Geometry: final body of the model. Coordinates: model frame, mm. Face numbers are marked on the shaded views. Round coordinates to 2 decimals unless told otherwise and drop trailing zeros. Write each loop counter-clockwise with the first axis right and the second up, starting at its lowest first coordinate (ties: lowest second). Pieces come first, ordered by that corner, then holes. Notation, with made-up numbers: (79, 2) - (97, 2) arc R28 ccw to (97, 33) - close; hole circle Ø9 at (23, -2). An arc over 180 degrees is marked (long way). Write each question's results on one line, items separated by ' | '.
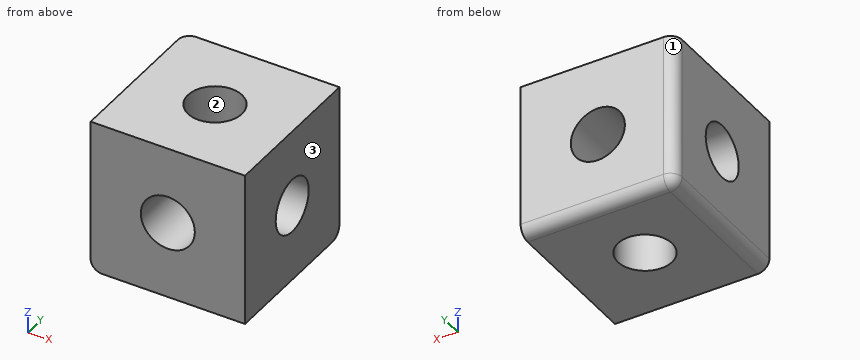
Autodesk Inventor part; units mm, degrees
ref_plane "YZ Plane" through (0, 0, 0) normal (1, 0, 0) x (0, 1, 0)
ref_plane "XZ Plane" through (0, 0, 0) normal (0, 1, 0) x (-1, 0, 0)
ref_plane "XY Plane" through (0, 0, 0) normal (0, 0, 1) x (1, 0, 0)
sketch "Sketch1" plane through (0, 0, 0) normal (0, 0, 1) x (1, 0, 0)
  line L0 (0, 0) -> (20, 0)
  line L1 (20, 0) -> (20, 20)
  line L2 (20, 20) -> (0, 20)
  line L3 (0, 20) -> (0, 0)
  circle A0 centre (10, 10) radius 3.5
  dimension "d0" = 20
  dimension "d1" = 20
  dimension "d2" = 7
extrude "Extrusion1" add sketch "Sketch1" along normal blind 20
sketch "Sketch2" plane through (20, 0, 0) normal (1, 0, 0) x (0, 0, -1)
  circle A0 centre (-10, 10) radius 3.5
  dimension "d5" = 7
extrude "Extrusion2" cut sketch "Sketch2" against normal blind 20
sketch "Sketch3" plane through (0, 0, 0) normal (0, -1, 0) x (1, 0, 0)
  circle A0 centre (10, 10) radius 3.5
  dimension "d8" = 7
extrude "Extrusion3" cut sketch "Sketch3" against normal blind 20
fillet "Fillet1" radius 1.5 3 edges at (0, 10, 0) (0, 20, 10) (10, 20, 0)
properties part number "Corner Profile"
Q1. Section query C-C, the plane y = 3.5. Return loops of the section in (x, z).
Answer block:
outline: (0, 1.5) arc R1.5 ccw to (1.5, 0) - (20, 0) - (20, 20) - (0, 20) - close; hole circle Ø7 at (10, 10)
Q2. Section query B-B, the plane z = 10. Return loops of the section in (x, y).
Answer block:
outline: (0, 0) - (6.5, 0) - (6.5, 6.5) - (0, 6.5) - close; (0, 13.5) - (6.5, 13.5) - (6.5, 20) - (1.5, 20) arc R1.5 ccw to (0, 18.5) - close; (13.5, 0) - (20, 0) - (20, 6.5) - (13.5, 6.5) - close; (13.5, 13.5) - (20, 13.5) - (20, 20) - (13.5, 20) - close
Q3. Ray query, line 1 along Y through (x, z) = (10, 14.75). Return the intervals inside material, ascending.
Answer block:
line 1: 0 to 6.5, 13.5 to 20
Q4. Mould query, pull axis Y, two halves, no side actions, for the marked faces 1, 2 and 3. Classes: pulls with the +Y half, pulls with the -Y half, needs draft (parallel to the pull), parting line crosses it, or undercut.
Answer block:
face 1: pulls with the +Y half | face 2: undercut | face 3: needs draft
Q5. Section query D-D, the plane x = 3. Return loops of the section in (y, z), plus the area to 3 significant figures.
Answer block:
outline: (0, 0) - (18.5, 0) arc R1.5 ccw to (20, 1.5) - (20, 20) - (0, 20) - close; hole circle Ø7 at (10, 10) | area: 361 mm2
Q6. Section query A-A, the plane y = 10. Return loops of the section in (x, z), plus the area to 3 significant figures.
Answer block:
outline: (0, 1.5) arc R1.5 ccw to (1.5, 0) - (6.5, 0) - (6.5, 6.5) - (0, 6.5) - close; (0, 13.5) - (6.5, 13.5) - (6.5, 20) - (0, 20) - close; (13.5, 0) - (20, 0) - (20, 6.5) - (13.5, 6.5) - close; (13.5, 13.5) - (20, 13.5) - (20, 20) - (13.5, 20) - close | area: 169 mm2
